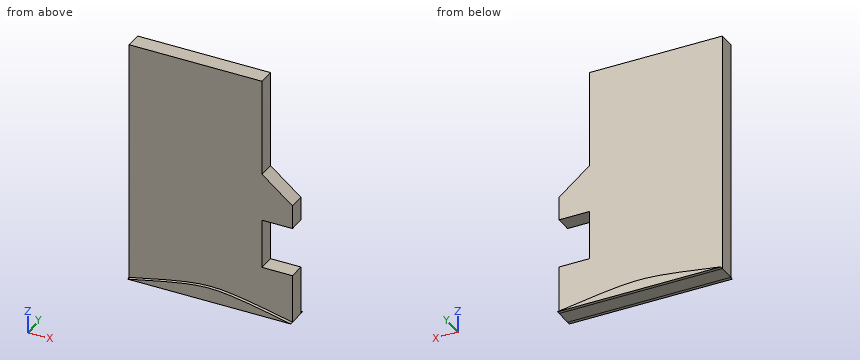
Autodesk Fusion 360 part; units mm, degrees
sketch "草图1" plane through (0, 0, 0) normal (0, 1, 0) x (1, 0, 0)
  line L0 (0, 0) -> (10, 0)
  line L1 (8.1421, -15) -> (0, -15)
  line L2 (0, -15) -> (0, 0)
  line L3 (8.1421, -15) -> (8.1421, -9)
  line L4 (8.1421, -9) -> (10, -7.5)
  line L5 (10, -6.0419) -> (8.1421, -6.0419)
  line L6 (8.1421, -6.0419) -> (8.1421, -3)
  line L7 (8.1421, -3) -> (10, -3)
  line L8 (10, 0) -> (10, -3)
  line L9 (10, -6.0419) -> (10, -7.5)
  dimension "d1" = 10
  dimension "d2" = 15
extrude "拉伸1" add sketch "草图1" along normal blind 1
sketch "草图2" plane through (0, 0, 0) normal (0, -1, 0) x (1, 0, 0)
  line L0 (8.1421, 3) -> (8.1421, 6.0419)
  line L1 (8.1421, 6.0419) -> (10, 6.0419)
  line L2 (10, 6.0419) -> (10, 7.5)
  line L3 (10, 7.5) -> (8.1421, 9)
  line L4 (8.1421, 9) -> (8.1421, 15)
  line L5 (8.1421, 15) -> (0, 15)
  line L6 (0, 15) -> (0, 0)
  line L7 (0, 0) -> (10, 0)
  line L8 (10, 0) -> (10, 3)
  line L9 (10, 3) -> (8.1421, 3)
  spline S0 degree 2 poles (0, 0) (5, 1.1516) (10, 0) knots 0 0 0 1.014809 1.014809 1.014809 weights 1 3 1
extrude "拉伸2" add sketch "草图2" along normal blind 0.2 contours L7 S0
sketch "草图3" plane through (0, 1, 0) normal (0, 1, 0) x (-1, 0, 0)
  line L0 (-8.1421, 6.0419) -> (-8.1421, 3)
  line L1 (-8.1421, 3) -> (-10, 3)
  line L2 (-10, 3) -> (-10, 0)
  line L3 (-10, 0) -> (0, 0)
  line L4 (0, 0) -> (0, 15)
  line L5 (0, 15) -> (-8.1421, 15)
  line L6 (-8.1421, 15) -> (-8.1421, 9)
  line L7 (-8.1421, 9) -> (-10, 7.5)
  line L8 (-10, 7.5) -> (-10, 6.0419)
  line L9 (-10, 6.0419) -> (-8.1421, 6.0419)
  spline S0 degree 2 poles (-10, 0) (-5, 0.809) (0, 0) knots 0 0 0 1.007336 1.007336 1.007336 weights 1 3 1
extrude "拉伸3" add sketch "草图3" along normal blind 0.2 contours L3 S0
Verification items for the finished model (mm, model axes). Coordinates: 2 decimals unless noted, no trailing zeros. Order: outer loops, then holes, each group sorted by start corner. A loop starts at its lowest first (then second) coordinate and runs counter-clockwise, first axis right, second up. Notation, with made-up numbers: (-24.75, 49) -> (17.25, 49) arc R19 cw to (17.25, 69) -> close; hole circle Ø9 at (30, 36.5). An arc over 180 degrees is marked (long way). Use CSV: the item, a comma, the result in double quotes. Start each with the question number.
Q1. Section check C-C, the plane z = 7.25. Record the cut outline in (x, y), and give its area (3 significant figures).
Q2. Thickness scan on line 1 along X through (y, z) = (0.95, 10.25); line 2 along Y through (x, z) = (4, 1.25); line 3 along Z through (x, y) = (8.25, 0.6). Record the ranges inside material, lowest first.
Q3. Depth check by flat-ended pin: P1, Ø0.8, axis at y = 0.5, z = 11.5, coming from the +X side; P2, Ø5, axis at x = 7, z = 6, coming from the -Y side; P3, Ø1, axis at x = 7, z = 9, coming from the +Y side. Enter the tip coordinate at first touch or a pass-through.
Q4. Section check A-A, the plane y = 0.85. Record the cut outline in (x, z), and give its area (3 significant figures).
Q5. Section check B-B, the plane z = 12. Record the cut outline in (x, y).
Returned:
1,outline,"(0, 0) -> (10, 0) -> (10, 1) -> (0, 1) -> close"
1,area,"10.0 mm^2"
2,line 1,"x = 0 to 8.14"
2,line 2,"y = 0 to 1"
2,line 3,"z = 0 to 3, 6.04 to 8.91"
3,P1,"stops at x = 8.14"
3,P2,"stops at y = 0"
3,P3,"stops at y = 1"
4,outline,"(0, 0) -> (10, 0) -> (10, 3) -> (8.14, 3) -> (8.14, 6.04) -> (10, 6.04) -> (10, 7.5) -> (8.14, 9) -> (8.14, 15) -> (0, 15) -> close"
4,area,"132 mm^2"
5,outline,"(0, 0) -> (8.14, 0) -> (8.14, 1) -> (0, 1) -> close"
